Build history of the part. All positions in model axes, mm. A direction names the side the tool comes from. Round coordinates to 2 decimals unless told otherwise and drop trailing zeros. Order: outer loops, then holes, each group sorted by start corner. A loop starts at its lowest first (then second) coordinate and runs counter-clockwise, first axis right, second up. Notation, with made-up numbers: (87, -24) - (93, -24) arc R32 cw to (93, 11) - close; hole circle Ø7 at (5, -19). An arc over 180 degrees is marked (long way). One line per question, with ' | ' between items. Start each with the question number.
from build123d import *

# Parameters (mm, degrees)
SKETCH1_W                          = 28.2
SKETCH1_H                          = 28.2
BOSS_EXTRUDE1_DEPTH                = 44.5
M2_5X0_45_TAPPED_HOLE1_D           = 2.05
M2_5X0_45_TAPPED_HOLE1_DEPTH       = 6.4
M2_5X0_45_TAPPED_HOLE1_CSINK_D     = 3
M2_5X0_45_TAPPED_HOLE1_CSINK_ANGLE = 90
M2_5X0_45_TAPPED_HOLE1_TIP         = 0.615882135
SKETCH15_R                         = 11
BOSS_EXTRUDE2_DEPTH                = 2
SKETCH16_R                         = 2.5
BOSS_EXTRUDE3_DEPTH                = 18
CUT_EXTRUDE1_DEPTH                 = 15


with BuildPart() as part:
    # Sketch1 → Boss-Extrude1 (new body)
    with BuildSketch(Plane.XY):
        with Locations((14.1, 14.1)):
            Rectangle(SKETCH1_W, SKETCH1_H)
    extrude(amount=BOSS_EXTRUDE1_DEPTH)

    # M2.5x0.45 Tapped Hole1
    with Locations(Plane.XY.offset(44.5)):
        with Locations((25.6, 2.6), (25.6, 25.6), (2.6, 2.6), (2.6, 25.6)):
            CounterSinkHole(M2_5X0_45_TAPPED_HOLE1_D / 2, M2_5X0_45_TAPPED_HOLE1_CSINK_D / 2, depth=M2_5X0_45_TAPPED_HOLE1_DEPTH, counter_sink_angle=M2_5X0_45_TAPPED_HOLE1_CSINK_ANGLE)
            with Locations((0, 0, -(M2_5X0_45_TAPPED_HOLE1_DEPTH + M2_5X0_45_TAPPED_HOLE1_TIP / 2))):  # 118° drill point
                Cone(0, M2_5X0_45_TAPPED_HOLE1_D / 2, M2_5X0_45_TAPPED_HOLE1_TIP, mode=Mode.SUBTRACT)

    # Sketch15 → Boss-Extrude2 (add)
    with BuildSketch(Plane.XY.offset(44.5)):
        with Locations((14.1, 14.1)):
            Circle(SKETCH15_R)
    extrude(amount=BOSS_EXTRUDE2_DEPTH)

    # Sketch16 → Boss-Extrude3 (add)
    with BuildSketch(Plane.XY.offset(46.5)):
        with Locations((14.1, 14.1)):
            Circle(SKETCH16_R)
    extrude(amount=BOSS_EXTRUDE3_DEPTH)

    # Sketch17 → Cut-Extrude1 (cut)
    with BuildSketch(Plane.XY.offset(64.5)):
        with BuildLine():
            Line((13.010275264, 16.35), (13.010275264, 11.85))
            ThreePointArc((13.010275264, 11.85), (11.6, 14.1), (13.010275264, 16.35))
        make_face()
    extrude(amount=-CUT_EXTRUDE1_DEPTH, mode=Mode.SUBTRACT)


solid = part.part
Item 1: Slice it at A-A (y = 14.1). Write the cut outline in (x, z).
Item 2: 3-axis set-ups, long thin cutter, end or side, ignore diameter. For faces 4 (the face through (12, 14, 49.5)), 5 (the face through (24.65, 25.21, 41.02)), 6 (the face through (14, 0, 22)): which of +Z, -Z, +X, -X, +Y, -Y reach the whole face in a straight line?
Item 3: Pin check, flat tips, straight feed: pin 1 (2.5 mm diameter, centred on x = 2.6, y = 2.6, fed in from +Z); pin 2 (1.5 mm diameter, centred on x = 12.5, y = 24, fed in from +Z); pin 3 (4 mm diameter, centred on x = 13, z = 48, fed in from +Y). Stop position of each tip, or through.
Item 4: Wall check: line 1 along Y through (x, z) = (25.6, 42.1) (3 decimals); line 2 along Z through (x, y) = (13.25, 17.5). Give the ranges that are in metal, low to high. Write a range as [from, to].
Item 5: Pull direction Y, two halves, no side cores. Call faces 1 (the face through (8, 24, 44.5)), 2 (the face through (16.41, 13.14, 55.37)), 3 (the face through (25.696, 25.75, 37.591)): released by +Y, released by -Y, zero draft, split by the parting line, or undercut.
Item 6: Slice it at D-D (y = 9.5). Write the cut outline in (x, z), plus the area to 3 significant figures.
Item 7: Slice it at B-B (x = 14.1). Write the cut outline in (y, z).
Item 8: Slice it at C-C (z = 54). Write the cut outline in (x, y).
A:
1) outline: (0, 0) - (28.2, 0) - (28.2, 44.5) - (25.1, 44.5) - (25.1, 46.5) - (16.6, 46.5) - (16.6, 64.5) - (13.01, 64.5) - (13.01, 49.5) - (11.6, 49.5) - (11.6, 46.5) - (3.1, 46.5) - (3.1, 44.5) - (0, 44.5) - close
2) face 4: +Z, -X, +Y, -Y | face 5: +Z | face 6: +Z, -Z, +X, -X, -Y
3) pin 1: z = 44.25 | pin 2: z = 46.5 | pin 3: y = 25.1
4) line 1: [0, 1.575], [3.625, 24.575], [26.625, 28.2] | line 2: [0, 46.5]
5) face 1: zero draft | face 2: split by the parting line | face 3: undercut
6) outline: (0, 0) - (28.2, 0) - (28.2, 44.5) - (24.09, 44.5) - (24.09, 46.5) - (4.11, 46.5) - (4.11, 44.5) - (0, 44.5) - close | area: 1,290 mm^2
7) outline: (0, 0) - (28.2, 0) - (28.2, 44.5) - (25.1, 44.5) - (25.1, 46.5) - (16.6, 46.5) - (16.6, 64.5) - (11.6, 64.5) - (11.6, 46.5) - (3.1, 46.5) - (3.1, 44.5) - (0, 44.5) - close
8) outline: (13.01, 11.85) arc R2.5 ccw (long way) to (13.01, 16.35) - close
